Verification items for the finished model (mm, model axes). Give positions to 0.01 mm unless a question says otherwise; leave off trailing zeros. Write each loop counter-clockwise with the first axis right and the second up, starting at its lowest first coordinate (ties: lowest second). Pieces come first, ordered by that corner, then holes.
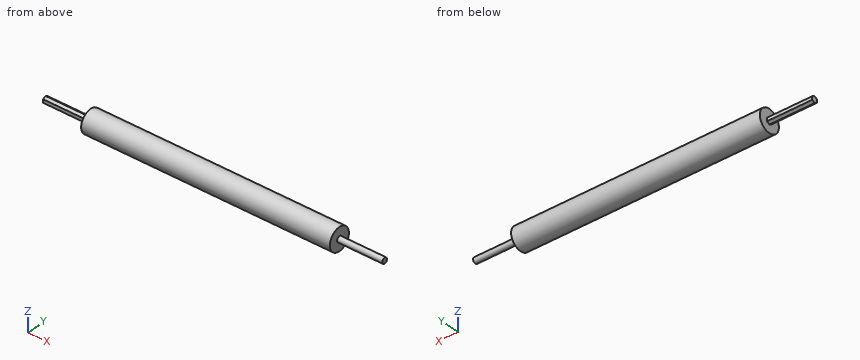
from build123d import *

# Parameters (mm, degrees)
F0_R     = 25.4
F1_DEPTH = 558.8
F2_R     = 6.35
F3_DEPTH = 101.6
F5_DEPTH = 101.6


with BuildPart() as f1:
    # F0 (on Right) → F1 (new body)
    with BuildSketch(Plane.YZ):
        Circle(F0_R)
    extrude(amount=F1_DEPTH)

    # F2 (on face) → F3 (join)
    with BuildSketch(Plane.YZ.offset(558.8)):
        Circle(F2_R)
    extrude(amount=F3_DEPTH)

    # F4 (on face) → F5 (join)
    with BuildSketch(Plane(origin=(0, 0, 0), x_dir=(0, -1, 0), z_dir=(-1, 0, 0))):
        Polygon((0.205691, -7.329463), (6.450346, -3.486598), (6.244656, 3.842865), (-0.205691, 7.329463), (-6.450346, 3.486598), (-6.244656, -3.842865), align=None)
    extrude(amount=F5_DEPTH)


solid = f1.part
Item 1: Sectioned sample at B-B on y = 18. Record the cut outline in (x, z), then the cut area to 3 significant figures.
Answer key:
outline: (0, -17.92) - (558.8, -17.92) - (558.8, 17.92) - (0, 17.92) - close
area: 20,000 mm2
Item 2: Scan lines: line 1 along X through (y, z) = (13, -5); line 2 along Y through (x, z) = (515.5, 2.5); line 3 along Y through (x, z) = (-2, 2). Record each from-to range of solid material in increasing order.
Answer key:
line 1: x = 0 to 558.8
line 2: y = -25.28 to 25.28
line 3: y = -6.3 to 6.41
Item 3: Sectioned sample at C-C on y = -17. Record the cut outline in (x, z).
Answer key:
outline: (0, -18.87) - (558.8, -18.87) - (558.8, 18.87) - (0, 18.87) - close
Item 4: Depth check by flat-ended pin: pin 1 (12 mm diameter, centred on y = -10.5, z = 3, fed in from +X); pin 2 (1 mm diameter, centred on x = 269, z = -10, fed in from +Y); pin 3 (5 mm diameter, centred on y = 17, z = 4, fed in from -X); pin 4 (1.5 mm diameter, centred on x = 327, y = -15.5, fed in from +Z). Enter the tip coordinate at first touch or a pass-through.
Answer key:
pin 1: stops at x = 660.4
pin 2: stops at y = 23.56
pin 3: stops at x = 0
pin 4: stops at z = 20.68
Item 5: Sectioned sample at A-A on x = 267.5. Record the cut outline in (y, z), then the cut area to 3 significant figures.
Answer key:
outline: circle Ø50.8 at (0, 0)
area: 2,030 mm2
